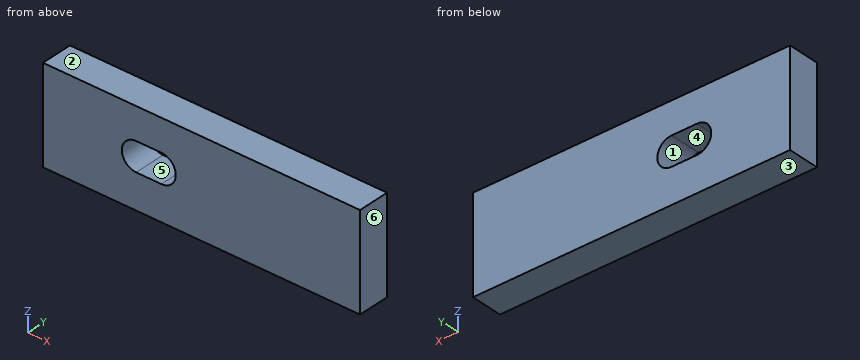
from build123d import *

# Parameters (mm, degrees)
F0_W     = 200
F0_H     = 60
F1_DEPTH = 20


with BuildPart() as f1:
    # F0 (on Front) → F1 (new body)
    with BuildSketch(Plane.XZ):
        with Locations((-12.351252, -25.980778)):
            Rectangle(F0_W, F0_H)
        with BuildLine():
            Line((-53.61577, -16.063345), (-37.61577, -16.063345))
            ThreePointArc((-37.61577, -16.063345), (-28.61577, -25.063345), (-37.61577, -34.063345))
            Line((-37.61577, -34.063345), (-53.61577, -34.063345))
            ThreePointArc((-53.61577, -34.063345), (-62.61577, -25.063345), (-53.61577, -16.063345))
        make_face(mode=Mode.SUBTRACT)
    extrude(amount=F1_DEPTH)


solid = f1.part
Read the model definition and answer for the solid it produces. Units are mm, in the model's axes. Face numbers are marked on the shaded views. A direction names the side the tool comes from. Round coordinates to 2 decimals unless told otherwise and drop trailing zeros. Loops run counter-clockwise (first coordinate to the right, second up) from the corner with the lowest first, then second, coordinate; pieces in that order, holes last.
Q1. Determine the mould class of the marked faces 3, 4, 5 and 6 for opening direction X: released by +X, released by -X, zero draft, split by the parting line, or undercut.
Q2. Section B-B on z = -22 is taken. Write down the section's boundary in (x, y).
Q3. Consider probe 1 along Z at (x, y) = (-32, -7); probe 2 along X at (y, z) = (-12, -22.5). Determine where each line is inside the solid, lowest interval first.
Q4. Which of the six approach directions +Z, -Z, +X, -X, +Y, -Y give full straight-line access (tool end or side, diameter ignored) to the marked faces 1 and 2?
Q5. Section A-A on y = -4.5 is taken. Write down the section's boundary in (x, z), and give its area (3 significant figures).
Output:
1. face 3: zero draft
1. face 4: undercut
1. face 5: undercut
1. face 6: released by +X
2. outline: (-112.35, -20) - (-62.08, -20) - (-62.08, 0) - (-112.35, 0) - close; (-29.15, -20) - (87.65, -20) - (87.65, 0) - (-29.15, 0) - close
3. probe 1: z = -55.98 to -32.1, -18.03 to 4.02
3. probe 2: x = -112.35 to -62.24, -28.99 to 87.65
4. face 1: +Y, -Y
4. face 2: +Z, +X, -X, +Y, -Y
5. outline: (-112.35, -55.98) - (87.65, -55.98) - (87.65, 4.02) - (-112.35, 4.02) - close; hole (-53.62, -34.06) - (-37.62, -34.06) arc R9 ccw to (-37.62, -16.06) - (-53.62, -16.06) arc R9 ccw to start
5. area: 11,500 mm2
